from build123d import *

# Parameters (mm, degrees)
SKETCH1_R           = 6.5
SKETCH1_R_2         = 3.57
SKETCH1_R_3         = 3
SKETCH1_R_4         = 1.5875
BOSS_EXTRUDE1_DEPTH = 10
SKETCH1_3_R         = 3.57
SKETCH1_3_R_2       = 3
SKETCH1_3_R_3       = 1.5875
BOSS_EXTRUDE2_DEPTH = 11.557
SKETCH1_4_R         = 3
SKETCH1_4_R_2       = 1.5875
BOSS_EXTRUDE3_DEPTH = 17
SKETCH1_5_R         = 1.5875
BOSS_EXTRUDE4_DEPTH = 30.5816
SKETCH2_R           = 0.35
BOSS_EXTRUDE5_DEPTH = 10


with BuildPart() as part:
    # Sketch1 → Boss-Extrude1 (new body)
    # profile 1 of 4: a face of its own
    with BuildSketch(Plane.XY):
        Circle(SKETCH1_R)
        Circle(SKETCH1_R_2, mode=Mode.SUBTRACT)
    # profile 2 of 4: a face of its own
    with BuildSketch(Plane.XY):
        Circle(SKETCH1_R_2)
        Circle(SKETCH1_R_3, mode=Mode.SUBTRACT)
    # profile 3 of 4: a face of its own
    with BuildSketch(Plane.XY):
        Circle(SKETCH1_R_3)
        Circle(SKETCH1_R_4, mode=Mode.SUBTRACT)
    # profile 4 of 4: a face of its own
    with BuildSketch(Plane.XY):
        Circle(SKETCH1_R_4)
    extrude(amount=BOSS_EXTRUDE1_DEPTH)

    # Sketch1_3 → Boss-Extrude2 (add)
    # profile 1 of 3: a face of its own
    with BuildSketch(Plane.XY):
        Circle(SKETCH1_3_R)
        Circle(SKETCH1_3_R_2, mode=Mode.SUBTRACT)
    # profile 2 of 3: a face of its own
    with BuildSketch(Plane.XY):
        Circle(SKETCH1_3_R_2)
        Circle(SKETCH1_3_R_3, mode=Mode.SUBTRACT)
    # profile 3 of 3: a face of its own
    with BuildSketch(Plane.XY):
        Circle(SKETCH1_3_R_3)
    extrude(amount=BOSS_EXTRUDE2_DEPTH)

    # Sketch1_4 → Boss-Extrude3 (add)
    # profile 1 of 2: a face of its own
    with BuildSketch(Plane.XY):
        Circle(SKETCH1_4_R)
        Circle(SKETCH1_4_R_2, mode=Mode.SUBTRACT)
    # profile 2 of 2: a face of its own
    with BuildSketch(Plane.XY):
        Circle(SKETCH1_4_R_2)
    extrude(amount=BOSS_EXTRUDE3_DEPTH)

    # Sketch1_5 → Boss-Extrude4 (add)
    with BuildSketch(Plane.XY):
        Circle(SKETCH1_5_R)
    extrude(amount=BOSS_EXTRUDE4_DEPTH)

    # Sketch2 → Boss-Extrude5 (add)
    with BuildSketch(Plane(origin=(0, 0, 0), x_dir=(-1, 0, 0), z_dir=(0, 0, -1))):
        with Locations(Location((-2.5, 2.5, 0), (0, 0, 180))):
            Circle(SKETCH2_R)
        with Locations(Location((2.5, 2.5, 0), (0, 0, 180))):
            Circle(SKETCH2_R)
        with Locations(Location((2.5, -2.5, 0), (0, 0, 180))):
            Circle(SKETCH2_R)
        with Locations(Location((-2.5, -2.5, 0), (0, 0, 180))):
            Circle(SKETCH2_R)
    extrude(amount=BOSS_EXTRUDE5_DEPTH)


solid = part.part
Part model, mm, in its own coordinate system. A direction names the side the tool comes from. Coordinates: 2 decimals unless noted, no trailing zeros. Order: outer loops, then holes, each group sorted by start corner. A loop starts at its lowest first (then second) coordinate and runs counter-clockwise, first axis right, second up. Notation, with made-up numbers: M 14.25,60 L 51.25,60 A22 cw 51.25,84 Z; hole C -22.75,68 d2. An arc over 180 degrees is marked long. Use a Markdown table: item, result.
(1) Cut at C-C on z = 14.5. Write the cut outline in (x, y).
A:
| item | result |
|---|---|
| outline | C 0,0 d6 |
(2) Cut at D-D on z = 23. Write the cut outline in (x, y) (1 decimal), then the cut area to 3 significant figures.
A:
| item | result |
|---|---|
| outline | C 0,0 d3.2 |
| area | 7.92 mm^2 |
(3) Tool access for faces 1 (the cylindrical face through (-0.34, -1.55, 23.7)), 2 (the flat face through (0, 0, 30.582)): list every direction of +Z, -Z, +X, -X, +Y, -Y with a clear straight run to the whole face (end or side of a thin tool).
A:
| item | result |
|---|---|
| face 1 | +Z |
| face 2 | +Z, +X, -X, +Y, -Y |
(4) Flat gauge pins, fed straight in: pin 1 (1.5 mm diameter, centred on x = 2.5, y = -2, fed in from +Z); pin 2 (3 mm diameter, centred on x = 3.5, y = -5, fed in from +Z); pin 3 (1 mm diameter, centred on x = -1.5, y = 4, fed in from -Z). Where does each tip first touch, or does it go through?
A:
| item | result |
|---|---|
| pin 1 | stops at z = 17 |
| pin 2 | stops at z = 10 |
| pin 3 | stops at z = 0 |
(5) Probe L1, parallel to Z at x = -4, y = -2.75; L2, parallel to Y at x = 0, z = 19; L3, parallel to Z at x = -2.25, y = -1.5. List the from-to ranges inside material, lowest first.
A:
| item | result |
|---|---|
| L1 | z = 0 to 10 |
| L2 | y = -1.59 to 1.59 |
| L3 | z = 0 to 17 |
(6) Cut at A-A on x = 0. Write the cut outline in (y, z).
A:
| item | result |
|---|---|
| outline | M -6.5,0 L 6.5,0 L 6.5,10 L 3.57,10 L 3.57,11.56 L 3,11.56 L 3,17 L 1.59,17 L 1.59,30.58 L -1.59,30.58 L -1.59,17 L -3,17 L -3,11.56 L -3.57,11.56 L -3.57,10 L -6.5,10 Z |
